Print and shaded views of the part. All mm, measured from the part's lowest x, y and z. A direction names the side the tool comes from. Give positions to 0.01 mm unless a question says otherwise; leave off trailing zeros. Loops run counter-clockwise (first coordinate to the right, second up) from the corner with the lowest first, then second, coordinate; pieces in that order, holes last. Notation, with made-up numbers: M -4,-12.75 L 46,-12.75 A25 cw 46,20.25 Z; hole C -39,50.25 d4. An arc over 180 degrees is marked long. Put each result on its own line as item: value. Start each with the question number.
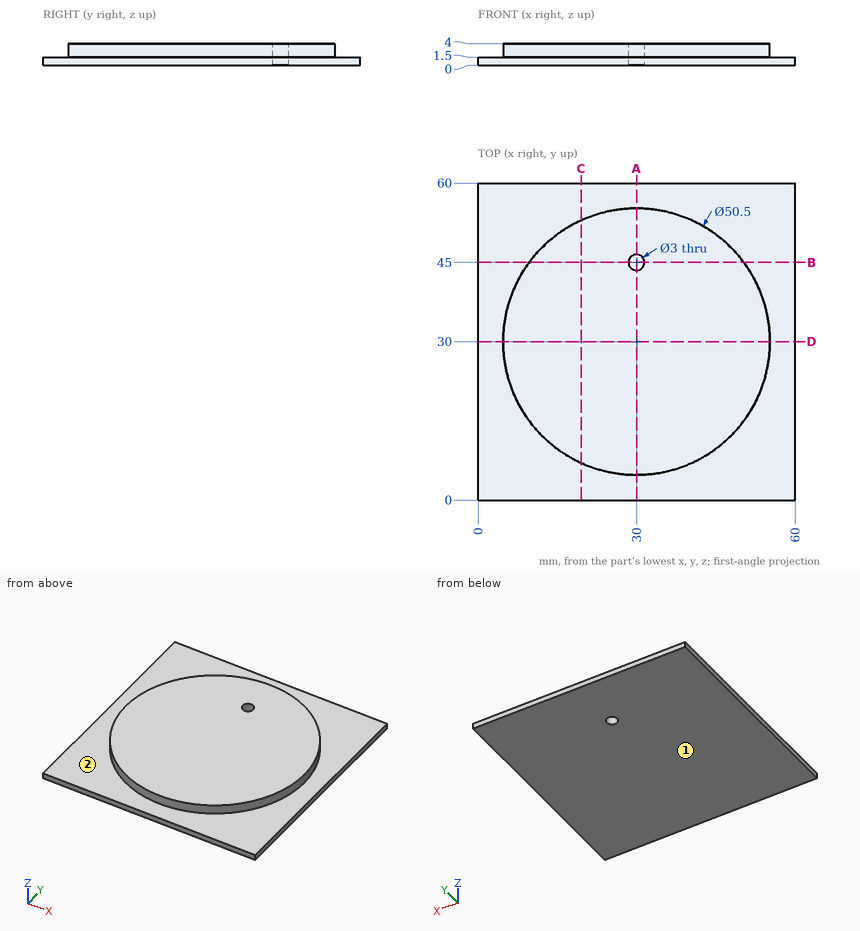
1) Band-saw the part on B-B on y = 45. Give the cut face in (x, z).
2) Band-saw the part on D-D on y = 30. Give the cut face in (x, z).
3) Band-saw the part on C-C on x = 19.5. Give the cut face in (y, z).
4) Wall check: L1, parallel to Y at x = 30, z = 1.3; L2, parallel to X at y = 30, z = 3.35; L3, parallel to Y at x = 30, z = 2.7. Give the ranges that are in metal, low to high.
5) Pin check, flat tips, straight feed: pin 1 Ø1.5 at (x, z) = (44, 2.5) entering from +Y; pin 2 Ø2 at (x, z) = (27.5, 3) entering from +Y; pin 3 Ø8 at (x, y) = (21, 33.5) entering from -Z. Stop position of each tip, or through.
6) Band-saw the part on A-A on x = 30. Give the cut face in (y, z), then the cut area to 3 significant figures.
7) Which spindle directions (+Z, -Z, +X, -X, +Y, -Y) get a long thin tool onto all of the face, cutting with end or side? Do the marked faces 1 and 2. Say none if no direction does.
Evaluation:
1. outline: M 0,0 L 28.5,0 L 28.5,4 L 9.69,4 L 9.69,1.5 L 0,1.5 Z; M 31.5,0 L 60,0 L 60,1.5 L 50.31,1.5 L 50.31,4 L 31.5,4 Z
2. outline: M 0,0 L 60,0 L 60,1.5 L 55.25,1.5 L 55.25,4 L 4.75,4 L 4.75,1.5 L 0,1.5 Z
3. outline: M 0,0 L 60,0 L 60,1.5 L 52.96,1.5 L 52.96,4 L 7.04,4 L 7.04,1.5 L 0,1.5 Z
4. L1: 0 to 43.5, 46.5 to 60
4. L2: 4.75 to 55.25
4. L3: 4.75 to 43.5, 46.5 to 55.25
5. pin 1: y = 51.49
5. pin 2: y = 55.21
5. pin 3: z = 0
6. outline: M 0,0 L 43.5,0 L 43.5,4 L 4.75,4 L 4.75,1.5 L 0,1.5 Z; M 46.5,0 L 60,0 L 60,1.5 L 55.25,1.5 L 55.25,4 L 46.5,4 Z
6. area: 204 mm2
7. face 1: -Z, +X, -X, +Y, -Y
7. face 2: +Z
